Work out the finished part from the listing and answer in its coordinate system (mm). Face numbers are marked on the shaded views. A direction names the side the tool comes from. Round coordinates to 2 decimals unless told otherwise and drop trailing zeros. Loops run counter-clockwise (first coordinate to the right, second up) from the corner with the lowest first, then second, coordinate; pieces in that order, holes last.
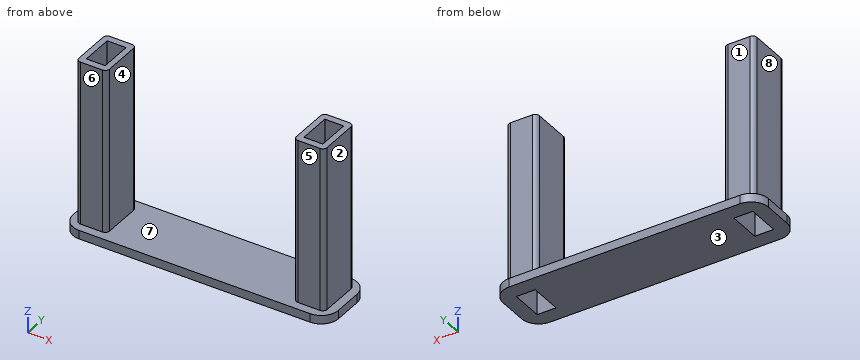
```python
from build123d import *

# Parameters (mm, degrees)
F0_W     = 78.0796
F0_H     = 18.5801
F1_DEPTH = 2.54
F2_W     = 8.99922
F2_H     = 13.5001
F2_W_2   = 8.999221
F3_DEPTH = 48.26
F4_R     = 5.08
F5_R     = 1.27
F6_W     = 5.55625
F6_H     = 9.525
F7_DEPTH = 76.2
F8_W     = 5.55625
F8_H     = 9.525
F9_DEPTH = 76.2


with BuildPart() as f1:
    # F0 (on Top) → F1 (new body)
    with BuildSketch(Plane.XY):
        Rectangle(F0_W, F0_H)
    extrude(amount=F1_DEPTH)

    # F2 (on face) → F3 (join)
    with BuildSketch(Plane.XY.offset(2.54)):
        with Locations((32.00019, 0)):
            Rectangle(F2_W, F2_H)
        with Locations((-32.000189, 0)):
            Rectangle(F2_W_2, F2_H)
    extrude(amount=F3_DEPTH)

    # F4
    f4_edges = [f1.edges().sort_by_distance(p)[0] for p in [
        (39.0398, 9.29005, 1.27),
        (39.0398, -9.29005, 1.27),
        (-39.0398, -9.29005, 1.27),
        (-39.0398, 9.29005, 1.27),
    ]]
    fillet(f4_edges, radius=F4_R)

    # F5
    f5_edges = [f1.edges().sort_by_distance(p)[0] for p in [
        (36.4998, 6.75005, 26.67),
        (36.4998, -6.75005, 26.67),
        (27.50058, -6.75005, 26.67),
        (27.50058, 6.75005, 26.67),
        (-27.500579, -6.75005, 26.67),
        (-36.4998, -6.75005, 26.67),
        (-36.4998, 6.75005, 26.67),
        (-27.500579, 6.75005, 26.67),
    ]]
    fillet(f5_edges, radius=F5_R)

    # F6 (on face) → F7 (cut)
    with BuildSketch(Plane.XY.offset(50.8)):
        with Locations((32.00019, 0)):
            Rectangle(F6_W, F6_H)
    extrude(amount=-F7_DEPTH, mode=Mode.SUBTRACT)

    # F8 (on face) → F9 (cut)
    with BuildSketch(Plane.XY.offset(50.8)):
        with Locations((-32.000189, 0)):
            Rectangle(F8_W, F8_H)
    extrude(amount=-F9_DEPTH, mode=Mode.SUBTRACT)


solid = f1.part
```
1. Consider probe 1 along X at (y, z) = (2.75, 39.5); probe 2 along Y at (x, z) = (33.5, 16.5); probe 3 along Z at (x, y) = (-3, -2.75). Determine where each line is inside the solid, lowest interval first.
Answer key:
probe 1: x = -36.5 to -34.78, -29.22 to -27.5, 27.5 to 29.22, 34.78 to 36.5
probe 2: y = -6.75 to -4.76, 4.76 to 6.75
probe 3: z = 0 to 2.54
2. Find section B-B (z = 17.5). Write down the section's boundary in (x, y).
Answer key:
outline: (-36.5, -5.48) arc R1.27 ccw to (-35.23, -6.75) - (-28.77, -6.75) arc R1.27 ccw to (-27.5, -5.48) - (-27.5, 5.48) arc R1.27 ccw to (-28.77, 6.75) - (-35.23, 6.75) arc R1.27 ccw to (-36.5, 5.48) - close; (27.5, -5.48) arc R1.27 ccw to (28.77, -6.75) - (35.23, -6.75) arc R1.27 ccw to (36.5, -5.48) - (36.5, 5.48) arc R1.27 ccw to (35.23, 6.75) - (28.77, 6.75) arc R1.27 ccw to (27.5, 5.48) - close; hole (-34.78, -4.76) - (-29.22, -4.76) - (-29.22, 4.76) - (-34.78, 4.76) - close; hole (29.22, -4.76) - (34.78, -4.76) - (34.78, 4.76) - (29.22, 4.76) - close
3. Given pin 1 (3 mm diameter, centred on x = -32, z = 20, fed in from +Y); pin 2 (7.5 mm diameter, centred on y = -2.5, z = 16, fed in from -X); pin 3 (10 mm diameter, centred on y = -1.5, z = 32, fed in from +X), each flat-ended and moving along its own axis, determine where each tip first touches the part or whether it passes through.
Answer key:
pin 1: stops at y = 6.75
pin 2: stops at x = -36.5
pin 3: stops at x = 36.5
4. Determine the mould class of the marked faces 6, 7 and 8 for opening direction X: +X half, -X half, draft (parallel to the pull), parting line (faces both ways), or undercut.
Answer key:
face 6: draft
face 7: undercut
face 8: -X half
5. Which of the six approach directions +Z, -Z, +X, -X, +Y, -Y give full straight-line access (tool end or side, diameter ignored) to the marked faces 1, 2, 3, 4 and 5?
Answer key:
face 1: +Z, +X, -X, +Y
face 2: +Z, +X, +Y, -Y
face 3: -Z, +X, -X, +Y, -Y
face 4: +Z, +Y, -Y
face 5: +Z, +X, -X, -Y
6. Find section D-D (y = -8). Write down the section's boundary in (x, z).
Answer key:
outline: (-37.34, 0) - (37.34, 0) - (37.34, 2.54) - (-37.34, 2.54) - close
7. Find section A-A (y = 1). Write down the section's boundary in (x, z), then the cut area to 3 significant figures.
Answer key:
outline: (-39.04, 0) - (-34.78, 0) - (-34.78, 50.8) - (-36.5, 50.8) - (-36.5, 2.54) - (-39.04, 2.54) - close; (-29.22, 0) - (29.22, 0) - (29.22, 50.8) - (27.5, 50.8) - (27.5, 2.54) - (-27.5, 2.54) - (-27.5, 50.8) - (-29.22, 50.8) - close; (34.78, 0) - (39.04, 0) - (39.04, 2.54) - (36.5, 2.54) - (36.5, 50.8) - (34.78, 50.8) - close
area: 502 mm2
8. Find section C-C (x = -9.5). Write down the section's boundary in (y, z).
Answer key:
outline: (-9.29, 0) - (9.29, 0) - (9.29, 2.54) - (-9.29, 2.54) - close
